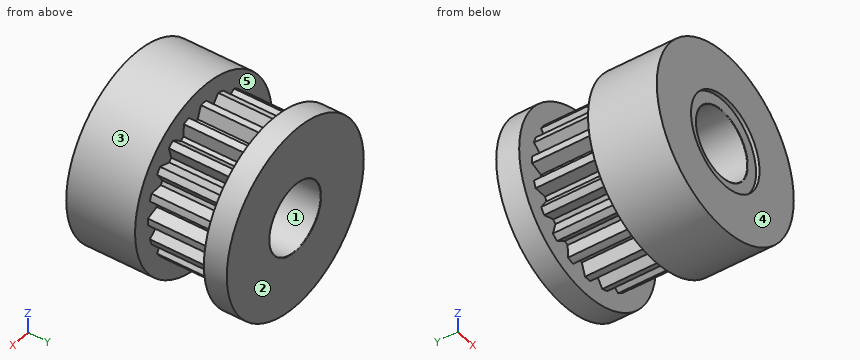
from build123d import *

# Parameters (mm, degrees)
SKETCH1_R           = 8
BOSS_EXTRUDE1_DEPTH = 6
BOSS_EXTRUDE2_DEPTH = 6
SKETCH3_R           = 8
BOSS_EXTRUDE3_DEPTH = 2
SKETCH4_R           = 3
CUT_EXTRUDE1_DEPTH  = 15
SKETCH5_R           = 4
CUT_EXTRUDE2_DEPTH  = 0.3
FILLET1_R           = 0.05


with BuildPart() as part:
    # Sketch1 → Boss-Extrude1 (new body)
    with BuildSketch(Plane(origin=(0, 0, 0), x_dir=(1, 0, 0), z_dir=(0, 1, 0))):
        Circle(SKETCH1_R)
    extrude(amount=-BOSS_EXTRUDE1_DEPTH)

    # Sketch2 → Boss-Extrude2 (add)
    with BuildSketch(Plane(origin=(0, 0, 0), x_dir=(1, 0, 0), z_dir=(0, 1, 0))):
        with BuildLine():
            Line((-0.305930382, 6.492796516), (-0.682763233, 5.457456767))
            ThreePointArc((-0.682763233, 5.457456767), (-0.860389558, 5.432285873), (-1.037100465, 5.401335263))
            Line((-1.037100465, 5.401335263), (-1.715427381, 6.269554123))
            ThreePointArc((-1.715427381, 6.269554123), (-2.008610463, 6.181867356), (-2.297341548, 6.080478749))
            Line((-2.297341548, 6.080478749), (-2.335793309, 4.979364379))
            ThreePointArc((-2.335793309, 4.979364379), (-2.496947749, 4.900535883), (-2.655445544, 4.81649343))
            Line((-2.655445544, 4.81649343), (-3.56886716, 5.43260409))
            ThreePointArc((-3.56886716, 5.43260409), (-3.82060414, 5.258610463), (-4.063872917, 5.072961356))
            Line((-4.063872917, 5.072961356), (-3.760179662, 4.013857112))
            ThreePointArc((-3.760179662, 4.013857112), (-3.889087297, 3.889087297), (-4.013857112, 3.760179662))
            Line((-4.013857112, 3.760179662), (-5.072961356, 4.063872917))
            ThreePointArc((-5.072961356, 4.063872917), (-5.258610463, 3.82060414), (-5.43260409, 3.56886716))
            Line((-5.43260409, 3.56886716), (-4.81649343, 2.655445544))
            ThreePointArc((-4.81649343, 2.655445544), (-4.900535883, 2.496947749), (-4.979364379, 2.335793309))
            Line((-4.979364379, 2.335793309), (-6.080478749, 2.297341548))
            ThreePointArc((-6.080478749, 2.297341548), (-6.181867356, 2.008610463), (-6.269554123, 1.715427381))
            Line((-6.269554123, 1.715427381), (-5.401335263, 1.037100465))
            ThreePointArc((-5.401335263, 1.037100465), (-5.432285873, 0.860389558), (-5.457456767, 0.682763233))
            Line((-5.457456767, 0.682763233), (-6.492796516, 0.305930382))
            ThreePointArc((-6.492796516, 0.305930382), (-6.5, 0), (-6.492796516, -0.305930382))
            Line((-6.492796516, -0.305930382), (-5.457456767, -0.682763233))
            ThreePointArc((-5.457456767, -0.682763233), (-5.432285873, -0.860389558), (-5.401335263, -1.037100465))
            Line((-5.401335263, -1.037100465), (-6.269554123, -1.715427381))
            ThreePointArc((-6.269554123, -1.715427381), (-6.181867356, -2.008610463), (-6.080478749, -2.297341548))
            Line((-6.080478749, -2.297341548), (-4.979364379, -2.335793309))
            ThreePointArc((-4.979364379, -2.335793309), (-4.900535883, -2.496947749), (-4.81649343, -2.655445544))
            Line((-4.81649343, -2.655445544), (-5.43260409, -3.56886716))
            ThreePointArc((-5.43260409, -3.56886716), (-5.258610463, -3.82060414), (-5.072961356, -4.063872917))
            Line((-5.072961356, -4.063872917), (-4.013857112, -3.760179662))
            ThreePointArc((-4.013857112, -3.760179662), (-3.889087297, -3.889087297), (-3.760179662, -4.013857112))
            Line((-3.760179662, -4.013857112), (-4.063872917, -5.072961356))
            ThreePointArc((-4.063872917, -5.072961356), (-3.82060414, -5.258610463), (-3.56886716, -5.43260409))
            Line((-3.56886716, -5.43260409), (-2.655445544, -4.81649343))
            ThreePointArc((-2.655445544, -4.81649343), (-2.496947749, -4.900535883), (-2.335793309, -4.979364379))
            Line((-2.335793309, -4.979364379), (-2.297341548, -6.080478749))
            ThreePointArc((-2.297341548, -6.080478749), (-2.008610463, -6.181867356), (-1.715427381, -6.269554123))
            Line((-1.715427381, -6.269554123), (-1.037100465, -5.401335263))
            ThreePointArc((-1.037100465, -5.401335263), (-0.860389558, -5.432285873), (-0.682763233, -5.457456767))
            Line((-0.682763233, -5.457456767), (-0.305930382, -6.492796516))
            ThreePointArc((-0.305930382, -6.492796516), (0, -6.5), (0.305930382, -6.492796516))
            Line((0.305930382, -6.492796516), (0.682763233, -5.457456767))
            ThreePointArc((0.682763233, -5.457456767), (0.860389558, -5.432285873), (1.037100465, -5.401335263))
            Line((1.037100465, -5.401335263), (1.715427381, -6.269554123))
            ThreePointArc((1.715427381, -6.269554123), (2.008610463, -6.181867356), (2.297341548, -6.080478749))
            Line((2.297341548, -6.080478749), (2.335793309, -4.979364379))
            ThreePointArc((2.335793309, -4.979364379), (2.496947749, -4.900535883), (2.655445544, -4.81649343))
            Line((2.655445544, -4.81649343), (3.56886716, -5.43260409))
            ThreePointArc((3.56886716, -5.43260409), (3.82060414, -5.258610463), (4.063872917, -5.072961356))
            Line((4.063872917, -5.072961356), (3.760179662, -4.013857112))
            ThreePointArc((3.760179662, -4.013857112), (3.889087297, -3.889087297), (4.013857112, -3.760179662))
            Line((4.013857112, -3.760179662), (5.072961356, -4.063872917))
            ThreePointArc((5.072961356, -4.063872917), (5.258610463, -3.82060414), (5.43260409, -3.56886716))
            Line((5.43260409, -3.56886716), (4.81649343, -2.655445544))
            ThreePointArc((4.81649343, -2.655445544), (4.900535883, -2.496947749), (4.979364379, -2.335793309))
            Line((4.979364379, -2.335793309), (6.080478749, -2.297341548))
            ThreePointArc((6.080478749, -2.297341548), (6.181867356, -2.008610463), (6.269554123, -1.715427381))
            Line((6.269554123, -1.715427381), (5.401335263, -1.037100465))
            ThreePointArc((5.401335263, -1.037100465), (5.432285873, -0.860389558), (5.457456767, -0.682763233))
            Line((5.457456767, -0.682763233), (6.492796516, -0.305930382))
            ThreePointArc((6.492796516, -0.305930382), (6.5, 0), (6.492796516, 0.305930382))
            Line((6.492796516, 0.305930382), (5.457456767, 0.682763233))
            ThreePointArc((5.457456767, 0.682763233), (5.432285873, 0.860389558), (5.401335263, 1.037100465))
            Line((5.401335263, 1.037100465), (6.269554123, 1.715427381))
            ThreePointArc((6.269554123, 1.715427381), (6.181867356, 2.008610463), (6.080478749, 2.297341548))
            Line((6.080478749, 2.297341548), (4.979364379, 2.335793309))
            ThreePointArc((4.979364379, 2.335793309), (4.900535883, 2.496947749), (4.81649343, 2.655445544))
            Line((4.81649343, 2.655445544), (5.43260409, 3.56886716))
            ThreePointArc((5.43260409, 3.56886716), (5.258610463, 3.82060414), (5.072961356, 4.063872917))
            Line((5.072961356, 4.063872917), (4.013857112, 3.760179662))
            ThreePointArc((4.013857112, 3.760179662), (3.889087297, 3.889087297), (3.760179662, 4.013857112))
            Line((3.760179662, 4.013857112), (4.063872917, 5.072961356))
            ThreePointArc((4.063872917, 5.072961356), (3.82060414, 5.258610463), (3.56886716, 5.43260409))
            Line((3.56886716, 5.43260409), (2.655445544, 4.81649343))
            ThreePointArc((2.655445544, 4.81649343), (2.496947749, 4.900535883), (2.335793309, 4.979364379))
            Line((2.335793309, 4.979364379), (2.297341548, 6.080478749))
            ThreePointArc((2.297341548, 6.080478749), (2.008610463, 6.181867356), (1.715427381, 6.269554123))
            Line((1.715427381, 6.269554123), (1.037100465, 5.401335263))
            ThreePointArc((1.037100465, 5.401335263), (0.860389558, 5.432285873), (0.682763233, 5.457456767))
            Line((0.682763233, 5.457456767), (0.305930382, 6.492796516))
            ThreePointArc((0.305930382, 6.492796516), (0, 6.5), (-0.305930382, 6.492796516))
        make_face()
    extrude(amount=BOSS_EXTRUDE2_DEPTH)

    # Sketch3 → Boss-Extrude3 (add)
    with BuildSketch(Plane(origin=(0, 6, 0), x_dir=(1, 0, 0), z_dir=(0, 1, 0))):
        Circle(SKETCH3_R)
    extrude(amount=BOSS_EXTRUDE3_DEPTH)

    # Sketch4 → Cut-Extrude1 (cut, through all)
    with BuildSketch(Plane.XZ.offset(6)):
        Circle(SKETCH4_R)
    extrude(amount=-CUT_EXTRUDE1_DEPTH, mode=Mode.SUBTRACT)

    # Sketch5 → Cut-Extrude2 (cut)
    with BuildSketch(Plane.XZ.offset(6)):
        Circle(SKETCH5_R)
    extrude(amount=-CUT_EXTRUDE2_DEPTH, mode=Mode.SUBTRACT)

    # Fillet1
    fillet1_edges = [part.edges().sort_by_distance(p)[0] for p in [
        (-3, 8, 0),
        (-3, -5.7, 0),
    ]]
    fillet(fillet1_edges, radius=FILLET1_R)


solid = part.part
Geometry check sheet. Reference: the model listing, model coordinates, mm. Face numbers are marked on the shaded views. A direction names the side the tool comes from. Give positions to 0.01 mm unless a question says otherwise; leave off trailing zeros. Write each loop counter-clockwise with the first axis right and the second up, starting at its lowest first coordinate (ties: lowest second). Pieces come first, ordered by that corner, then holes. Notation, with made-up numbers: (9.5, 44) - (37.5, 44) arc R35 cw to (37.5, 76) - close; hole circle Ø10 at (-1.75, 30). An arc over 180 degrees is marked (long way). Put each result on its own line as item: value.
1. Sectioned sample at D-D, the plane z = 4.5. Enter the section's corners in (x, y).
Ans:
outline: (-6.61, -6) - (6.61, -6) - (6.61, 0) - (3.9, 0) - (3.9, 6) - (6.61, 6) - (6.61, 8) - (-6.61, 8) - (-6.61, 6) - (-3.9, 6) - (-3.9, 0) - (-6.61, 0) - close
2. Thickness scan on line 1 (Y direction, x = -1.25, z = 5.75); line 2 (Z direction, x = 0, y = -5.9); line 3 (X direction, y = 5.25, z = -6). Record the ranges inside material, lowest first.
Ans:
line 1: y = -6 to 0, 6 to 8
line 2: z = -8 to -4, 4 to 8
line 3: x = -2.3 to -1.5, -0.49 to 0.49, 1.5 to 2.3
3. Go/stop test with flat-tipped pins: pin 1 (1 mm diameter, centred on x = 2.5, y = 2.5, fed in from -Z); pin 2 (2 mm diameter, centred on x = 3, y = -4, fed in from -Z); pin 3 (2 mm diameter, centred on x = -6, y = 4, fed in from +Z). Record where each tip stops, or that it passes through.
Ans:
pin 1: stops at z = -6.18
pin 2: stops at z = -7.75
pin 3: stops at z = 4.06
4. Draft check along X on the marked faces 1, 2 and 3. Enter one of: +X half, -X half, draft (parallel to the pull), parting line (faces both ways), or undercut.
Ans:
face 1: undercut
face 2: draft
face 3: parting line
5. Sectioned sample at A-A, the plane z = 0. Enter the section's corners in (x, y).
Ans:
outline: (-8, -6) - (-4, -6) - (-4, -5.7) - (-3.05, -5.7) arc R0.05 ccw to (-3, -5.65) - (-3, 7.95) arc R0.05 ccw to (-3.05, 8) - (-8, 8) - (-8, 6) - (-6.5, 6) - (-6.5, 0) - (-8, 0) - close; (3, -5.65) arc R0.05 ccw to (3.05, -5.7) - (4, -5.7) - (4, -6) - (8, -6) - (8, 0) - (6.5, 0) - (6.5, 6) - (8, 6) - (8, 8) - (3.05, 8) arc R0.05 ccw to (3, 7.95) - close
6. Set-up check for the marked faces 4 and 5: record each of +Z, -Z, +X, -X, +Y, -Y from which the full face is reachable in a straight line by a thin tool's end or side.
Ans:
face 4: +Z, -Z, +X, -X, -Y
face 5: none
7. Sectioned sample at B-B, the plane x = 0. Enter the section's corners in (y, z).
Ans:
outline: (-6, -8) - (0, -8) - (0, -6.5) - (6, -6.5) - (6, -8) - (8, -8) - (8, -3.05) arc R0.05 ccw to (7.95, -3) - (-5.65, -3) arc R0.05 ccw to (-5.7, -3.05) - (-5.7, -4) - (-6, -4) - close; (-6, 4) - (-5.7, 4) - (-5.7, 3.05) arc R0.05 ccw to (-5.65, 3) - (7.95, 3) arc R0.05 ccw to (8, 3.05) - (8, 8) - (6, 8) - (6, 6.5) - (0, 6.5) - (0, 8) - (-6, 8) - close
8. Sectioned sample at C-C, the plane y = -1. Enter the section's corners in (x, z).
Ans:
outline: circle Ø16 at (0, 0); hole circle Ø6 at (0, 0)
